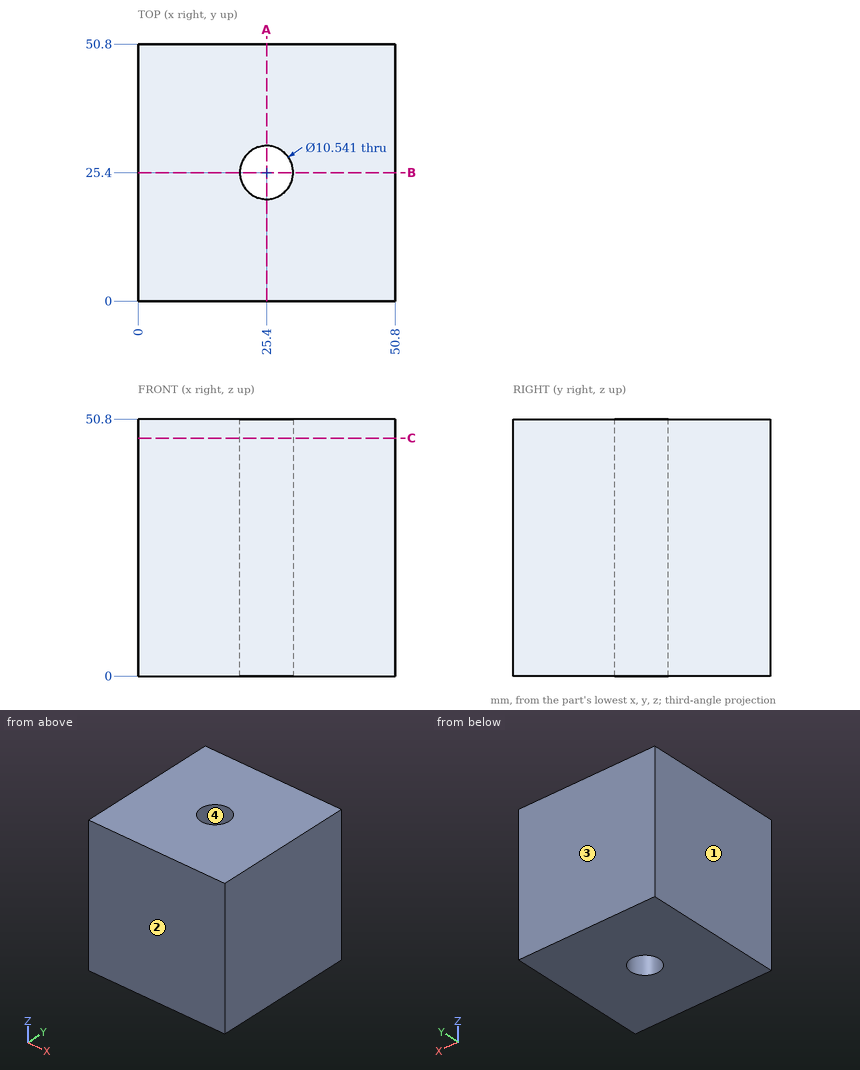
Here's the drawing with two shaded views (mm, measured from the low corner). I have some questions. Round coordinates to 2 decimals unless told otherwise and drop trailing zeros. Loops run counter-clockwise (first coordinate to the right, second up) from the corner with the lowest first, then second, coordinate; pieces in that order, holes last. Notation, with made-up numbers: M 4,73 L 18,73 A22 ccw 18,107 Z; hole C 60,4.25 d5. An arc over 180 degrees is marked long. Answer as CSV lines item,"result".
1) We'd pull the mould along Y, two halves only. Please class the marked faces 1, 2, 3 and 4: released by +Y, released by -Y, zero draft, split by the parting line, or undercut.
From the geometry:
face 1,"zero draft"
face 2,"released by -Y"
face 3,"released by +Y"
face 4,"undercut"
2) Imagine slicing it at A-A on x = 25.4. List the corners of the cut face in (y, z) for me, and give its area (3 significant figures).
From the geometry:
outline,"M 0,0 L 20.13,0 L 20.13,50.8 L 0,50.8 Z; M 30.67,0 L 50.8,0 L 50.8,50.8 L 30.67,50.8 Z"
area,"2,050 mm^2"
3) Imagine slicing it at C-C on z = 47. List the corners of the cut face in (x, y) for me, and give its area (3 significant figures).
From the geometry:
outline,"M 0,0 L 50.8,0 L 50.8,50.8 L 0,50.8 Z; hole C 25.4,25.4 d10.54"
area,"2,490 mm^2"
4) If I drill on probe 1 along Y at (x, z) = (25, 18); probe 2 along X at (y, z) = (29, 21), over which ranges is the centre line in solid material (lowest first)?
From the geometry:
probe 1,"0 to 20.14, 30.66 to 50.8"
probe 2,"0 to 21.55, 29.25 to 50.8"
5) For pin 1 Ø10 at (y, z) = (23.5, 25) entering from -X; pin 2 Ø6.5 at (x, y) = (25.4, 25.4) entering from -Z, each with a flat end and sliding along its axis, tell me the tip position at first contact or that it passes through.
From the geometry:
pin 1,"x = 0"
pin 2,"through"
